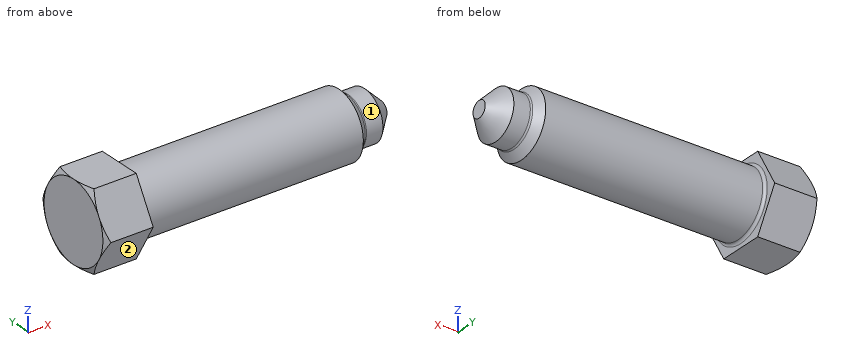
```python
from build123d import *

# Parameters (mm, degrees)
BASEHEAD_DEPTH = 14
HEADFILLET_R   = 0.8
POINTFILLET_R  = 0.8


with BuildPart() as part:
    # HexSke → BaseHead (new body)
    with BuildSketch(Plane(origin=(0, 0, 0), x_dir=(0, 0, -1), z_dir=(1, 0, 0))):
        Polygon((12, 6.92820323), (12, -6.92820323), (0, -13.856406461), (-12, -6.92820323), (-12, 6.92820323), (0, 13.856406461), align=None)
    extrude(amount=BASEHEAD_DEPTH)

    # BodySke → BaseBody (revolve)
    with BuildSketch(Plane.XY, mode=Mode.PRIVATE) as basebody_sk:
        Polygon((0, 0), (94, 0), (94, 2.5), (89, 7.5), (83.64, 7.5), (81.14, 10), (0, 10), align=None)
    revolve(basebody_sk.sketch.rotate(Axis((0, 0, 0), (1, 0, 0)), 90), axis=Axis((0, 0, 0), (1, 0, 0)))

    # Sketch3 → HeadChamfer (revolve, cut)
    with BuildSketch(Plane.XY):
        Polygon((0, 12), (3.958548116, 18.856406461), (3.958548116, 23.856406461), (-10, 23.856406461), (-10, 12), align=None)
    revolve(axis=Axis((0, 0, 0), (1, 0, 0)), mode=Mode.SUBTRACT)

    # HeadFillet
    headfillet_edges = [part.edges().sort_by_distance(p)[0] for p in [
        (14, 0, -10),
    ]]
    fillet(headfillet_edges, radius=HEADFILLET_R)

    # PointFillet
    pointfillet_edges = [part.edges().sort_by_distance(p)[0] for p in [
        (83.64, 0, -7.5),
    ]]
    fillet(pointfillet_edges, radius=POINTFILLET_R)


solid = part.part
```
Read the model definition and answer for the solid it produces. Units are mm, in the model's axes. Face numbers are marked on the shaded views. A direction names the side the tool comes from. Give positions to 0.01 mm unless a question says otherwise; leave off trailing zeros. Order: outer loops, then holes, each group sorted by start corner. A loop starts at its lowest first (then second) coordinate and runs counter-clockwise, first axis right, second up.
(1) For the marked faces 1 and 2, determine the directions among +Z, -Z, +X, -X, +Y, -Y from which every point of the face is accessible in a straight line to the end or side of a thin tool.
(2) Straight lines are drawn through the part: L1, parallel to Y at x = 85, z = -0.5; L2, parallel to X at y = -9, z = 6.75; L3, parallel to Z at x = 79, y = -0.5. For each, find the intervals that lie inside material, in ascending order.
(3) Given pin 1 (2 mm diameter, centred on x = 21, y = -1, fed in from +Z); pin 2 (5 mm diameter, centred on x = 17.5, y = -9.5, fed in from -Z); pin 3 (6 mm diameter, centred on x = 20.5, y = -1, fed in from -Z); pin 4 (12 mm diameter, centred on y = -0.5, z = 1, fed in from -X), each flat-ended and moving along its own axis, determine where each tip first touches the part or whether it passes through.
(4) Find section A-A (x = 38). Give the vertices of the cut face in (y, z), plus the area to 3 significant figures.
Result sheet:
1. face 1: +X
1. face 2: -Z, +X, -X, -Y
2. L1: y = -7.48 to 7.48
2. L2: x = 0 to 14
2. L3: z = -9.99 to 9.99
3. pin 1: stops at z = 10
3. pin 2: stops at z = -7.14
3. pin 3: stops at z = -10
3. pin 4: stops at x = 0
4. outline: circle Ø20 at (0, 0)
4. area: 314 mm2
